Print and shaded views of the part. All mm, measured from the part's lowest x, y and z. A direction names the side the tool comes from. Coordinates: 2 decimals unless noted, no trailing zeros. Order: outer loops, then holes, each group sorted by start corner. A loop starts at its lowest first (then second) coordinate and runs counter-clockwise, first axis right, second up. Notation, with made-up numbers: (61.5, 15) -> (101.5, 15) arc R26 ccw to (101.5, 37) -> close; hole circle Ø2 at (-10, 57). An arc over 180 degrees is marked (long way). Return JSON: item names as keys, results as strings. Group by question number.
1) Probe line 1 (X direction, y = 86, z = 2.05); line 2 (X direction, y = 102, z = 1.95); line 3 (Z direction, x = 107, y = 78). List the from-to ranges inside material, lowest first.
2) Cut at A-A (y = 102). Write the cut outline in (x, z), and give its area (3 significant figures).
3) Which spindle directions (+Z, -Z, +X, -X, +Y, -Y) get a long thin tool onto all of the face, cutting with end or side? Do the marked faces 1, 2, 3 and 4. Say none if no direction does.
4) Cut at D-D (z = 9). Write the cut outline in (x, y), and give its area (3 significant figures).
5) Cut at C-C (y = 18.5). Write the cut outline in (x, z), and give its area (3 significant figures).
6) Flat gauge pins, fed straight in: pin 1 (2 mm diameter, centred on x = 69.5, z = 7, fed in from +Y); pin 2 (3 mm diameter, centred on x = 40, y = 86, fed in from +Z); pin 3 (1.6 mm diameter, centred on y = 11, z = 12.5, fed in from +X); pin 4 (10 mm diameter, centred on x = 38, y = 84, fed in from -Z). Where does each tip first touch, or does it go through?
7) Cut at B-B (x = 22). Write the cut outline in (y, z).
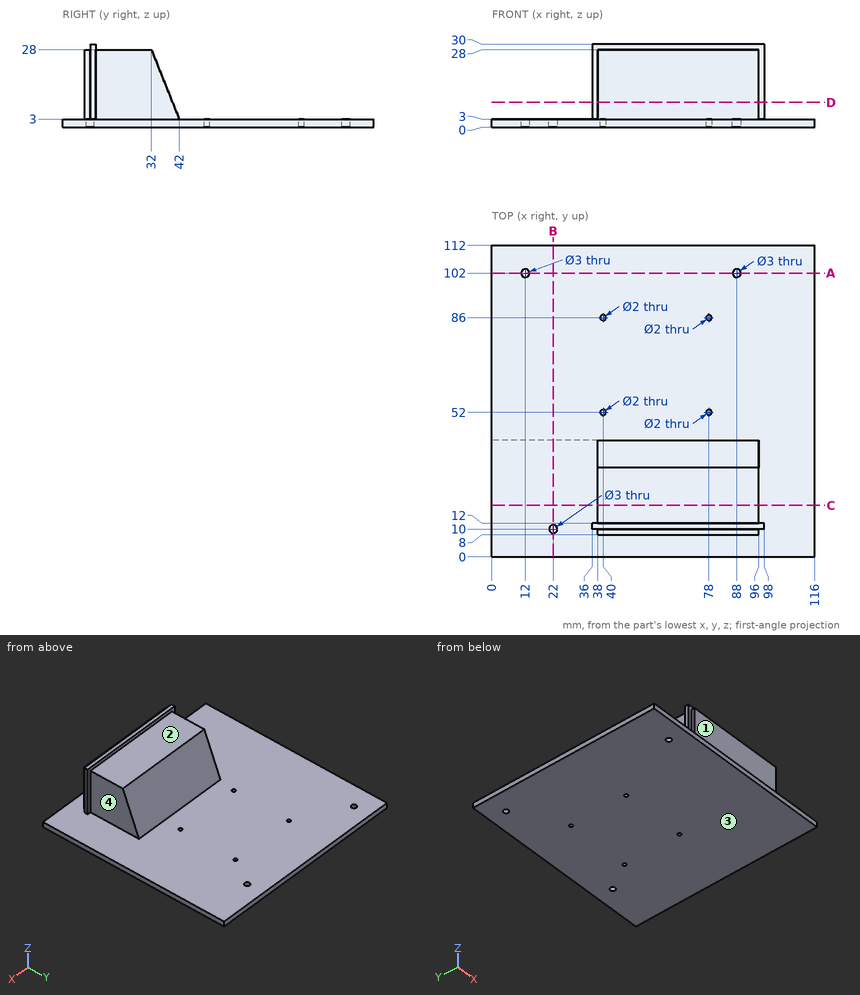
Answers below:
{
 "1": {"line 1": "x = 0 to 39, 41 to 77, 79 to 116", "line 2": "x = 0 to 10.5, 13.5 to 86.5, 89.5 to 116", "line 3": "z = 0 to 3"},
 "2": {"outline": "(0, 0) -> (10.5, 0) -> (10.5, 3) -> (0, 3) -> close; (13.5, 0) -> (86.5, 0) -> (86.5, 3) -> (13.5, 3) -> close; (89.5, 0) -> (116, 0) -> (116, 3) -> (89.5, 3) -> close", "area": "330 mm^2"},
 "3": {"face 1": "+Z, +X, -X, -Y", "face 2": "+Z, +X, -X, +Y", "face 3": "-Z, +X, -X, +Y, -Y", "face 4": "+Z, +X, +Y"},
 "4": {"outline": "(36, 10) -> (38, 10) -> (38, 8) -> (96, 8) -> (96, 10) -> (98, 10) -> (98, 12) -> (96, 12) -> (96, 39.6) -> (38, 39.6) -> (38, 12) -> (36, 12) -> close", "area": "1,840 mm^2"},
 "5": {"outline": "(0, 0) -> (116, 0) -> (116, 3) -> (96, 3) -> (96, 28) -> (38, 28) -> (38, 3) -> (0, 3) -> close", "area": "1,800 mm^2"},
 "6": {"pin 1": "stops at y = 40.8", "pin 2": "stops at z = 3", "pin 3": "stops at x = 98", "pin 4": "stops at z = 0"},
 "7": {"outline": "(0, 0) -> (8.5, 0) -> (8.5, 3) -> (0, 3) -> close; (11.5, 0) -> (112, 0) -> (112, 3) -> (11.5, 3) -> close"}
}
